Can you work these out from the model? Positions are in its coordinate system, mm. Coordinates: 2 decimals unless noted, no trailing zeros. Order: outer loops, then holes, each group sorted by start corner. A loop starts at its lowest first (then second) coordinate and runs counter-clockwise, first axis right, second up. Notation, with made-up numbers: (77.25, 72) -> (122.25, 72) arc R22 ccw to (122.25, 79) -> close; hole circle Ø9 at (47.25, -18). An arc over 180 degrees is marked (long way). Use a Markdown table: item, result. Add a question column.
1. Suppose I cut it at C-C, the plane y = 1.5. List the corners of the cut face in (x, z) for me, then the cut area to 3 significant figures.
2. Suppose I cut it at B-B, the plane z = 1.1. List the corners of the cut face in (x, y) for me, then the cut area to 3 significant figures.
3. Suppose I cut it at D-D, the plane x = -3.25. List the corners of the cut face in (y, z) for me.
4. Suppose I cut it at A-A, the plane x = -10.25. List the corners of the cut face in (y, z) for me.
5. We'd pull the mould along X, two halves only. Please class faces 1 (the cylindrical face through (19.75, 0.08, 0.74)), 2 (the cylindrical face through (-3.2, -2.5, 0.7)), 3 (the flat face through (2, 0, 0)): pulls with the +X half, pulls with the -X half, needs draft (parallel to the pull), parting line crosses it, or undercut.
6. If I drill on line 1 along Y through (x, z) = (-10.25, 0.4); line 2 along X through (y, z) = (-1, 0.2); line 3 along X through (y, z) = (-2.75, 0.95), over which ranges is the centre line in solid material (lowest first)? Write a range as from..to.
```python
from build123d import *

# Parameters (mm, degrees)
SKETCH1_R           = 2
BOSS_EXTRUDE1_DEPTH = 1.5


with BuildPart() as part:
    # Sketch1 → Boss-Extrude1 (new body)
    with BuildSketch(Plane.XY):
        with BuildLine():
            Line((-16.25, 3.5), (-4.25, 3.5))
            ThreePointArc((-4.25, 3.5), (-3.25, 2.5), (-2.25, 3.5))
            Line((-2.25, 3.5), (16.25, 3.5))
            ThreePointArc((16.25, 3.5), (19.75, 0), (16.25, -3.5))
            Line((16.25, -3.5), (-2.25, -3.5))
            ThreePointArc((-2.25, -3.5), (-3.25, -2.5), (-4.25, -3.5))
            Line((-4.25, -3.5), (-16.25, -3.5))
            Line((-16.25, -3.5), (-16.25, 3.5))
        make_face()
        with Locations((-10.25, 0)):
            Circle(SKETCH1_R, mode=Mode.SUBTRACT)
    extrude(amount=BOSS_EXTRUDE1_DEPTH)


solid = part.part
```
Worked out:
| question | item | result |
|---|---|---|
| 1 | outline | (-16.25, 0) -> (-11.57, 0) -> (-11.57, 1.5) -> (-16.25, 1.5) -> close; (-8.93, 0) -> (19.41, 0) -> (19.41, 1.5) -> (-8.93, 1.5) -> close |
| 1 | area | 49.5 mm² |
| 2 | outline | (-16.25, -3.5) -> (-4.25, -3.5) arc R1 cw to (-2.25, -3.5) -> (16.25, -3.5) arc R3.5 ccw to (16.25, 3.5) -> (-2.25, 3.5) arc R1 cw to (-4.25, 3.5) -> (-16.25, 3.5) -> close; hole circle Ø4 at (-10.25, 0) |
| 2 | area | 231 mm² |
| 3 | outline | (-2.5, 0) -> (2.5, 0) -> (2.5, 1.5) -> (-2.5, 1.5) -> close |
| 4 | outline | (-3.5, 0) -> (-2, 0) -> (-2, 1.5) -> (-3.5, 1.5) -> close; (2, 0) -> (3.5, 0) -> (3.5, 1.5) -> (2, 1.5) -> close |
| 5 | face 1 | pulls with the +X half |
| 5 | face 2 | undercut |
| 5 | face 3 | needs draft |
| 6 | line 1 | y = -3.5..-2, 2..3.5 |
| 6 | line 2 | x = -16.25..-11.98, -8.52..19.6 |
| 6 | line 3 | x = -16.25..-3.91, -2.59..18.42 |
